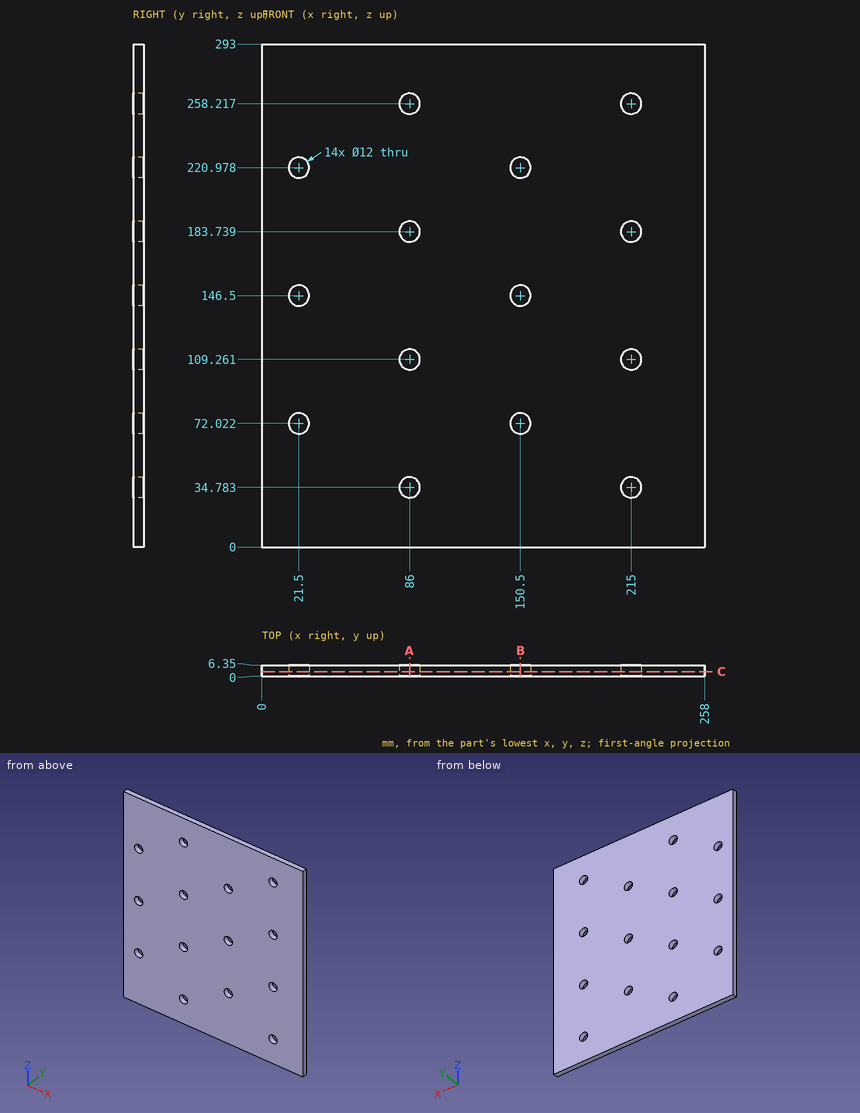
Source: three-view drawing plus pictorial views. Frame: mm from the lowest corner of the part. Coordinates: 2 decimals unless noted, no trailing zeros. Loops run counter-clockwise (first coordinate to the right, second up) from the corner with the lowest first, then second, coordinate; pieces in that order, holes last. Notation, with made-up numbers: (60.25, -37) -> (115.25, -37) arc R29 cw to (115.25, -1) -> close; hole circle Ø2 at (57.25, -19). An arc over 180 degrees is marked (long way). One line per item, written item: value.
(1) Cut plane B-B (x = 150.5). Output: boundary loops of the cut face in (y, z).
Answer below:
outline: (0, 0) -> (6.35, 0) -> (6.35, 66.02) -> (0, 66.02) -> close; (0, 78.02) -> (6.35, 78.02) -> (6.35, 140.5) -> (0, 140.5) -> close; (0, 152.5) -> (6.35, 152.5) -> (6.35, 214.98) -> (0, 214.98) -> close; (0, 226.98) -> (6.35, 226.98) -> (6.35, 293) -> (0, 293) -> close
(2) Cut plane C-C (y = 2.5). Give the number of separate pieces and of enclosed holes in the cut face, then the cut area to 3 significant figures.
Answer below:
separate pieces: 1
enclosed holes: 14
area: 74,000 mm2
(3) Cut plane A-A (x = 86). Output: boundary loops of the cut face in (y, z).
Answer below:
outline: (0, 0) -> (6.35, 0) -> (6.35, 28.78) -> (0, 28.78) -> close; (0, 40.78) -> (6.35, 40.78) -> (6.35, 103.26) -> (0, 103.26) -> close; (0, 115.26) -> (6.35, 115.26) -> (6.35, 177.74) -> (0, 177.74) -> close; (0, 189.74) -> (6.35, 189.74) -> (6.35, 252.22) -> (0, 252.22) -> close; (0, 264.22) -> (6.35, 264.22) -> (6.35, 293) -> (0, 293) -> close
(4) Ray query, line 1 along Z through (x, y) = (21, 0.75); line 2 along Z through (x, y) = (86, 2); line 3 along X through (y, z) = (3, 146.5). Return the intervals inside material, ascending.
Answer below:
line 1: z = 0 to 66.04, 78 to 140.52, 152.48 to 215, 226.96 to 293
line 2: z = 0 to 28.78, 40.78 to 103.26, 115.26 to 177.74, 189.74 to 252.22, 264.22 to 293
line 3: x = 0 to 15.5, 27.5 to 144.5, 156.5 to 258
